from build123d import *

# Parameters (mm, degrees)
ESBO_O1_R                = 2
ESBO_O1_R_2              = 2.086716092
ESBO_O1_R_3              = 2.086717953
RESSALTO_EXTRUS_O1_DEPTH = 8
ESBO_O4_R                = 1.65
CORTE_EXTRUS_O1_DEPTH    = 9


with BuildPart() as part:
    # Esboço1 → Ressalto-extrusão1 (new body)
    with BuildSketch(Plane.XY):
        Polygon((19.311716217, 92), (-19.311716217, 92), (-36.5, 70), (-36.5, 0), (-22.499999998, 0), (-22.499999998, 8.400000004), (22.499999998, 8.400000004), (22.499999998, 0), (36.5, 0), (36.5, 70), align=None)
        with Locations((0, 75)):
            Circle(ESBO_O1_R, mode=Mode.SUBTRACT)
        with Locations((-7, 83.3)):
            Circle(ESBO_O1_R, mode=Mode.SUBTRACT)
        with Locations((7, 83.3)):
            Circle(ESBO_O1_R, mode=Mode.SUBTRACT)
        with Locations((-29.2, 10)):
            Circle(ESBO_O1_R, mode=Mode.SUBTRACT)
        with Locations((29.2, 10)):
            Circle(ESBO_O1_R, mode=Mode.SUBTRACT)
        with Locations((-16, 56.354540575)):
            Circle(ESBO_O1_R_2, mode=Mode.SUBTRACT)
        with Locations((16, 56.354540575)):
            Circle(ESBO_O1_R_3, mode=Mode.SUBTRACT)
        Polygon((0, 47.257129716), (8.5, 47.257129716), (8.5, 23.917682695), (0, 23.917682695), (-8.5, 23.917682695), (-8.5, 47.257129716), align=None, mode=Mode.SUBTRACT)
    extrude(amount=RESSALTO_EXTRUS_O1_DEPTH)

    # Esboço4 → Corte-extrusão1 (cut, through all)
    with BuildSketch(Plane.XY.offset(8)):
        with Locations((-29.2, 66)):
            Circle(ESBO_O4_R)
        with Locations((-29.2, 53)):
            Circle(ESBO_O4_R)
        with Locations((29.2, 53)):
            Circle(ESBO_O4_R)
        with Locations((29.2, 66)):
            Circle(ESBO_O4_R)
    extrude(amount=-CORTE_EXTRUS_O1_DEPTH, mode=Mode.SUBTRACT)


solid = part.part
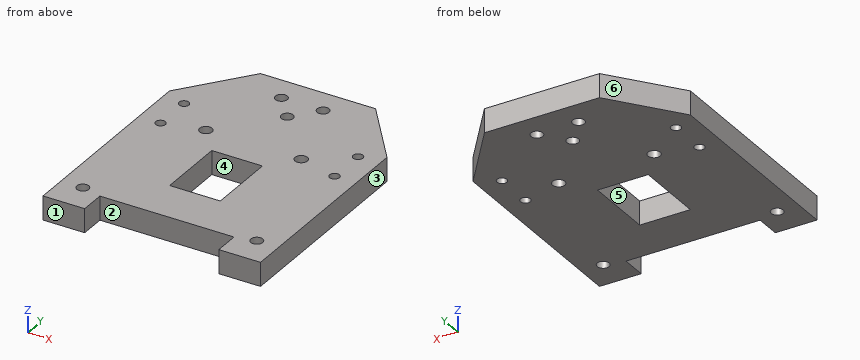
CAD build for the part. Positions are in the model's coordinates, mm. Face numbers are marked on the shaded views. A direction names the side the tool comes from. Give positions to 0.01 mm unless a question says otherwise; leave off trailing zeros. Loops run counter-clockwise (first coordinate to the right, second up) from the corner with the lowest first, then second, coordinate; pieces in that order, holes last. Notation, with made-up numbers: M 26.5,15.25 L 68.5,15.25 A20 ccw 68.5,53.25 Z; hole C -25.75,33.25 d3. An arc over 180 degrees is marked long. Write each question's results on one line, items separated by ' | '.
Q1. Band-saw the part on D-D on z = 5.75. Give the number of separate pieces and of enclosed holes in the cut face, and give its area (3 significant figures).
Geometry check:
separate pieces: 1 | enclosed holes: 12 | area: 5,440 mm²
Q2. Probe probe 1 along X at (y, z) = (51.5, 4.25); probe 2 along Y at (x, z) = (-29.2, 5.75); probe 3 along Y at (x, z) = (29, 0.75). List the from-to ranges inside material, lowest first.
Geometry check:
probe 1: x = -36.5 to -29.89, -28.51 to 28.51, 29.89 to 36.5 | probe 2: y = 0 to 8, 12 to 51.35, 54.65 to 64.35, 67.65 to 79.34 | probe 3: y = 0 to 8.01, 11.99 to 51.36, 54.64 to 64.36, 67.64 to 79.6
Q3. Which spindle directions (+Z, -Z, +X, -X, +Y, -Y) get a long thin tool onto all of the face, cutting with end or side? Do the marked faces 5 and 6. Say none if no direction does.
Geometry check:
face 5: +Z, -Z | face 6: +Z, -Z, -X, +Y
Q4. Band-saw the part on C-C on x = 29.2. Write the cut outline in (y, z).
Geometry check:
outline: M 0,0 L 8,0 L 8,8 L 0,8 Z; M 12,0 L 51.35,0 L 51.35,8 L 12,8 Z; M 54.65,0 L 64.35,0 L 64.35,8 L 54.65,8 Z; M 67.65,0 L 79.34,0 L 79.34,8 L 67.65,8 Z
Q5. Flat gauge pins, fed straight in: P1, Ø3.5, axis at x = -29.2, y = 10, coming from the -Z side; P2, Ø5, axis at x = 29.2, y = 10, coming from the +Z side; P3, Ø3, axis at x = -1.5, z = 3, coming from the -Y side. Where does each tip first touch, or does it go through?
Geometry check:
P1: passes through | P2: stops at z = 8 | P3: stops at y = 8.4
Q6. Mould opens along X. For the marked faces 1, 2, 3 and 4 say: pulls with the +X half, pulls with the -X half, needs draft (parallel to the pull), parting line crosses it, or undercut.
Geometry check:
face 1: needs draft | face 2: undercut | face 3: pulls with the +X half | face 4: undercut
Q7. Band-saw the part on B-B on y = 53. Write the cut outline in (x, z), and give its area (3 significant figures).
Geometry check:
outline: M -36.5,0 L -30.85,0 L -30.85,8 L -36.5,8 Z; M -27.55,0 L 27.55,0 L 27.55,8 L -27.55,8 Z; M 30.85,0 L 36.5,0 L 36.5,8 L 30.85,8 Z | area: 531 mm²
Q8. Band-saw the part on A-A on x = -7. Write the cut outline in (y, z), and give its area (3 significant figures).
Geometry check:
outline: M 8.4,0 L 23.92,0 L 23.92,8 L 8.4,8 Z; M 47.26,0 L 81.3,0 L 81.3,8 L 47.26,8 Z; M 85.3,0 L 92,0 L 92,8 L 85.3,8 Z | area: 450 mm²
